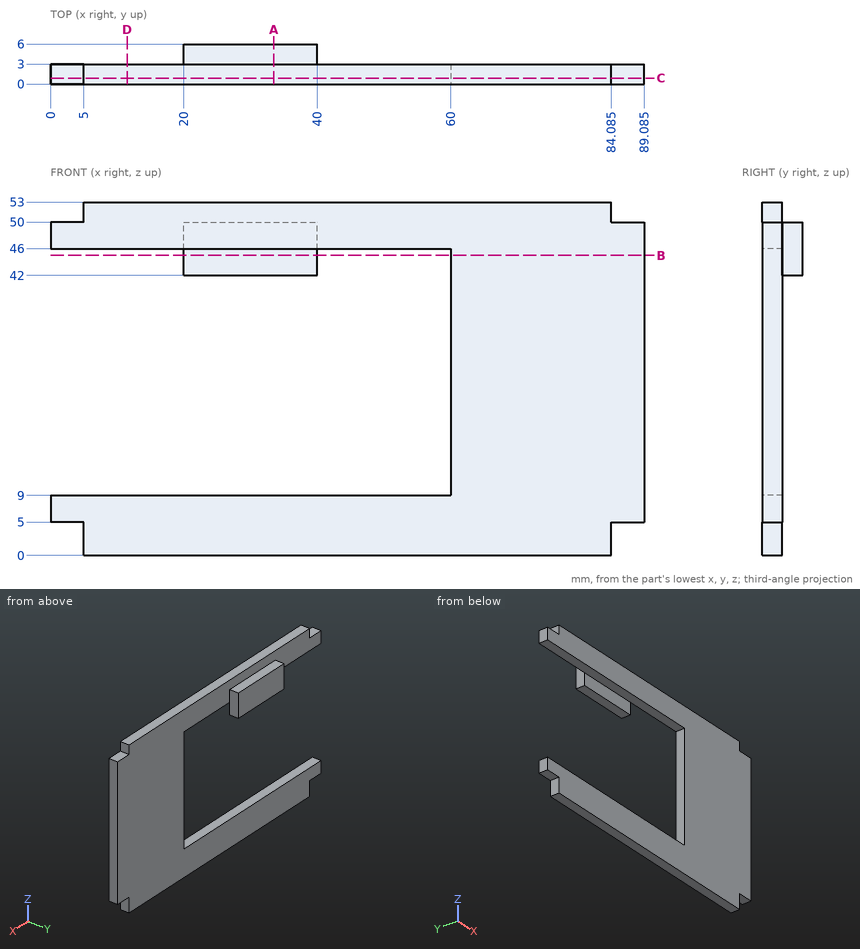
Could you check a few things on this drawing? It's one solid part, dimensions in mm from its lowest x, y, z. Round coordinates to 2 decimals unless told otherwise and drop trailing zeros. Write each loop counter-clockwise with the first axis right and the second up, starting at its lowest first coordinate (ties: lowest second). Pieces come first, ordered by that corner, then holes. Notation, with made-up numbers: M 29,-7.75 L 54,-7.75 A17 cw 54,6.25 Z; hole C 77.25,88 d2. An arc over 180 degrees is marked long. Answer as CSV lines item,"result". Start each with the question number.
1. I need wall thicknesses on probe 1 along Z at (x, y) = (19, 1.8); probe 2 along X at (y, z) = (3.2, 44.5); probe 3 along Y at (x, z) = (75, 11.5). Which ranges of each line are inside material? Lowest first, please.
2. Suppose I cut it at B-B on z = 45. Write out the boundary of the cut face in (x, y) (1 decimal).
3. Suppose I cut it at A-A on x = 33.5. Write out the boundary of the cut face in (y, z), then the cut area to 3 significant figures.
4. Suppose I cut it at D-D on x = 11.5. Write out the boundary of the cut face in (y, z).
5. Suppose I cut it at C-C on y = 0.9. Write out the boundary of the cut face in (x, z) (1 decimal), then the cut area to 3 significant figures.
6. I'm going to push flat-ended pins straight in: pin 1 Ø3.5 at (x, y) = (88, 1) entering from -Z; pin 2 Ø0.9 at (x, y) = (88, 1) entering from +Z; pin 3 Ø1 at (x, y) = (75, 5) entering from +Z; pin 4 Ø0.9 at (y, z) = (1, 2) entering from -X. Where does each tip first touch, or does it pass through?
Check result:
1,probe 1,"z = 0 to 9, 46 to 53"
1,probe 2,"x = 20 to 40"
1,probe 3,"y = 0 to 3"
2,outline,"M 20,3 L 40,3 L 40,6 L 20,6 Z; M 60,0 L 89.1,0 L 89.1,3 L 60,3 Z"
3,outline,"M 0,0 L 3,0 L 3,9 L 0,9 Z; M 0,46 L 3,46 L 3,42 L 6,42 L 6,50 L 3,50 L 3,53 L 0,53 Z"
3,area,"72.0 mm2"
4,outline,"M 0,0 L 3,0 L 3,9 L 0,9 Z; M 0,46 L 3,46 L 3,53 L 0,53 Z"
5,outline,"M 0,5 L 5,5 L 5,0 L 84.1,0 L 84.1,5 L 89.1,5 L 89.1,50 L 84.1,50 L 84.1,53 L 5,53 L 5,50 L 0,50 L 0,46 L 60,46 L 60,9 L 0,9 Z"
5,area,"2,420 mm2"
6,pin 1,"stops at z = 5"
6,pin 2,"stops at z = 50"
6,pin 3,"passes through"
6,pin 4,"stops at x = 5"
